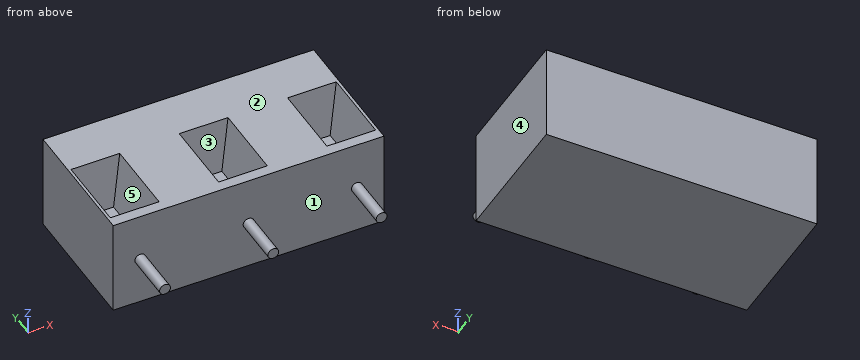
```python
from build123d import *

# Parameters (mm, degrees)
SKETCH1_W                    = 25
SKETCH1_H                    = 9
BOSS_EXTRUDE1_DEPTH          = 12.5
SKETCH2_R                    = 0.5
BOSS_EXTRUDE2_DEPTH          = 4.4
SKETCH3_W                    = 4.5
SKETCH3_H                    = 7
CUT_EXTRUDE1_DEPTH           = 4.4
CUT_EXTRUDE1_DRAFT           = -15
CUT_EXTRUDE1_PROFILE_2_DEPTH = 4.4
CUT_EXTRUDE1_PROFILE_2_DRAFT = -15
CUT_EXTRUDE1_PROFILE_3_DEPTH = 4.4
CUT_EXTRUDE1_PROFILE_3_DRAFT = -15


with BuildPart() as part:
    # Sketch1 → Boss-Extrude1 (new body)
    with BuildSketch(Plane(origin=(0, 0, 0), x_dir=(1, 0, 0), z_dir=(0, 1, 0))):
        Rectangle(SKETCH1_W, SKETCH1_H)
    extrude(amount=BOSS_EXTRUDE1_DEPTH)

    # Sketch2 → Boss-Extrude2 (add)
    with BuildSketch(Plane.XZ):
        with Locations(Location((0, 0, 0), (0, 0, 270))):
            Circle(SKETCH2_R)
        with Locations(Location((-10, 0, 0), (0, 0, 270))):
            Circle(SKETCH2_R)
        with Locations(Location((10, 0, 0), (0, 0, 270))):
            Circle(SKETCH2_R)
    extrude(amount=BOSS_EXTRUDE2_DEPTH)


with BuildPart() as cut_extrude1_tool:
    # Sketch3 → Cut-Extrude1 (with draft: the straight prism first)
    with BuildSketch(Plane.XY.offset(4.5)):
        with Locations((0, 4.5)):
            Rectangle(SKETCH3_W, SKETCH3_H)
    extrude(amount=-CUT_EXTRUDE1_DEPTH)
    # Cut-Extrude1: the draft: its side faces are tilted about the plane it starts from
    cut_extrude1_sides = [cut_extrude1_tool.faces().sort_by_distance(p)[0] for p in [
        (0, 1, 2.3),
        (2.25, 4.5, 2.3),
        (0, 8, 2.3),
        (-2.25, 4.5, 2.3),
    ]]
    draft(cut_extrude1_sides, Plane.XY.offset(4.5), CUT_EXTRUDE1_DRAFT)


with BuildPart() as part_1:
    add(part.part)

    # Cut-Extrude1: cut by cut_extrude1_tool
    add(cut_extrude1_tool.part, mode=Mode.SUBTRACT)


with BuildPart() as cut_extrude1_profile_2_tool:
    # Sketch3 → Cut-Extrude1 profile 2 (with draft: the straight prism first)
    with BuildSketch(Plane.XY.offset(4.5)):
        with Locations((10, 4.5)):
            Rectangle(SKETCH3_W, SKETCH3_H)
    extrude(amount=-CUT_EXTRUDE1_PROFILE_2_DEPTH)
    # Cut-Extrude1 profile 2: the draft: its side faces are tilted about the plane it starts from
    cut_extrude1_profile_2_sides = [cut_extrude1_profile_2_tool.faces().sort_by_distance(p)[0] for p in [
        (10, 1, 2.3),
        (12.25, 4.5, 2.3),
        (10, 8, 2.3),
        (7.75, 4.5, 2.3),
    ]]
    draft(cut_extrude1_profile_2_sides, Plane.XY.offset(4.5), CUT_EXTRUDE1_PROFILE_2_DRAFT)


with BuildPart() as part_2:
    add(part_1.part)

    # Cut-Extrude1 profile 2: cut by cut_extrude1_profile_2_tool
    add(cut_extrude1_profile_2_tool.part, mode=Mode.SUBTRACT)


with BuildPart() as cut_extrude1_profile_3_tool:
    # Sketch3 → Cut-Extrude1 profile 3 (with draft: the straight prism first)
    with BuildSketch(Plane.XY.offset(4.5)):
        with Locations((-10, 4.5)):
            Rectangle(SKETCH3_W, SKETCH3_H)
    extrude(amount=-CUT_EXTRUDE1_PROFILE_3_DEPTH)
    # Cut-Extrude1 profile 3: the draft: its side faces are tilted about the plane it starts from
    cut_extrude1_profile_3_sides = [cut_extrude1_profile_3_tool.faces().sort_by_distance(p)[0] for p in [
        (-10, 1, 2.3),
        (-7.75, 4.5, 2.3),
        (-10, 8, 2.3),
        (-12.25, 4.5, 2.3),
    ]]
    draft(cut_extrude1_profile_3_sides, Plane.XY.offset(4.5), CUT_EXTRUDE1_PROFILE_3_DRAFT)


with BuildPart() as part_3:
    add(part_2.part)

    # Cut-Extrude1 profile 3: cut by cut_extrude1_profile_3_tool
    add(cut_extrude1_profile_3_tool.part, mode=Mode.SUBTRACT)


solid = part_3.part
```
The listing builds one solid part. Answer for the finished solid, in the listing's coordinates (mm). Face numbers are marked on the shaded views. A direction names the side the tool comes from. Give positions to 0.01 mm unless a question says otherwise; leave off trailing zeros. Order: outer loops, then holes, each group sorted by start corner. A loop starts at its lowest first (then second) coordinate and runs counter-clockwise, first axis right, second up. Notation, with made-up numbers: (70, 84.25) - (125, 84.25) arc R22 cw to (125, 112.25) - close; hole circle Ø9 at (-38, 58.5). An arc over 180 degrees is marked (long way). Answer in a Markdown table with one row per item. Add a question column.
Q1. For a pull along Y with two mould halves and no side action, classify the marked faces 1, 2 and 3 as released by +Y, released by -Y, zero draft, split by the parting line, or undercut.
Q2. The part is cut by section D-D (z = -3.75). Determine the outline of the cut face in (x, y), then the cut area to 4 significant figures.
Q3. The part is cut by section A-A (z = 1.5). Determine the outline of the cut face in (x, y), then the cut area to 3 significant figures.
Q4. The part is cut by section C-C (y = -1.5). Determine the outline of the cut face in (x, z), then the cut area to 3 significant figures.
Q5. Which of the six approach directions +Z, -Z, +X, -X, +Y, -Y give full straight-line access (tool end or side, diameter ignored) to the marked faces 4 and 5?
Q6. Given P1, Ø2.5, axis at x = 4.5, z = -2, coming from the -Y side; P2, Ø0.6, axis at x = -10, y = 5, coming from the +Z side, each flat-ended and moving along its own axis, determine where each tip first touches the part or whether it passes through.
Q7. Find the intervals of material crossed by line 1 along X through (y, z) = (4.75, 2.75); line 2 along Y through (x, z) = (6.5, 2.5); line 3 along Y through (x, z) = (-10.5, 3.25), in increasing order. Write a range as [from, to].
Q8. The part is cut by section B-B (x = 10). Determine the outline of the cut face in (y, z), then the cut area to 3 significant figures.
Determined:
| question | item | result |
|---|---|---|
| 1 | face 1 | released by -Y |
| 1 | face 2 | zero draft |
| 1 | face 3 | undercut |
| 2 | outline | (-12.5, 0) - (12.5, 0) - (12.5, 12.5) - (-12.5, 12.5) - close |
| 2 | area | 312.5 mm² |
| 3 | outline | (-12.5, 0) - (12.5, 0) - (12.5, 12.5) - (-12.5, 12.5) - close; hole (-11.45, 1.8) - (-8.55, 1.8) - (-8.55, 7.2) - (-11.45, 7.2) - close; hole (-1.45, 1.8) - (1.45, 1.8) - (1.45, 7.2) - (-1.45, 7.2) - close; hole (8.55, 1.8) - (11.45, 1.8) - (11.45, 7.2) - (8.55, 7.2) - close |
| 3 | area | 266 mm² |
| 4 | outline | circle Ø1 at (-10, 0); circle Ø1 at (0, 0); circle Ø1 at (10, 0) |
| 4 | area | 2.36 mm² |
| 5 | face 4 | +Z, -Z, +X, +Y, -Y |
| 5 | face 5 | +Z |
| 6 | P1 | stops at y = 0 |
| 6 | P2 | stops at z = 0.1 |
| 7 | line 1 | x = [-12.5, -11.78], [-8.22, -1.78], [1.78, 8.22], [11.78, 12.5] |
| 7 | line 2 | y = [0, 12.5] |
| 7 | line 3 | y = [0, 1.33], [7.67, 12.5] |
| 8 | outline | (-4.4, -0.5) - (0, -0.5) - (0, -4.5) - (12.5, -4.5) - (12.5, 4.5) - (8, 4.5) - (6.82, 0.1) - (2.18, 0.1) - (1, 4.5) - (0, 4.5) - (0, 0.5) - (-4.4, 0.5) - close |
| 8 | area | 91.3 mm² |
